The drawing under review shows one solid part. Ordinate dimensions are in mm from its lowest x, y, z. A direction names the side the tool comes from. Give positions to 0.01 mm unless a question says otherwise; leave off trailing zeros. Write each loop counter-clockwise with the first axis right and the second up, starting at its lowest first coordinate (ties: lowest second). Pieces come first, ordered by that corner, then holes. Notation, with made-up numbers: M 89,-25 L 125,-25 A32 cw 125,10 Z; hole C 76,76 d8. An arc over 180 degrees is marked long. Write item = value, one per line. Start each with the question number.
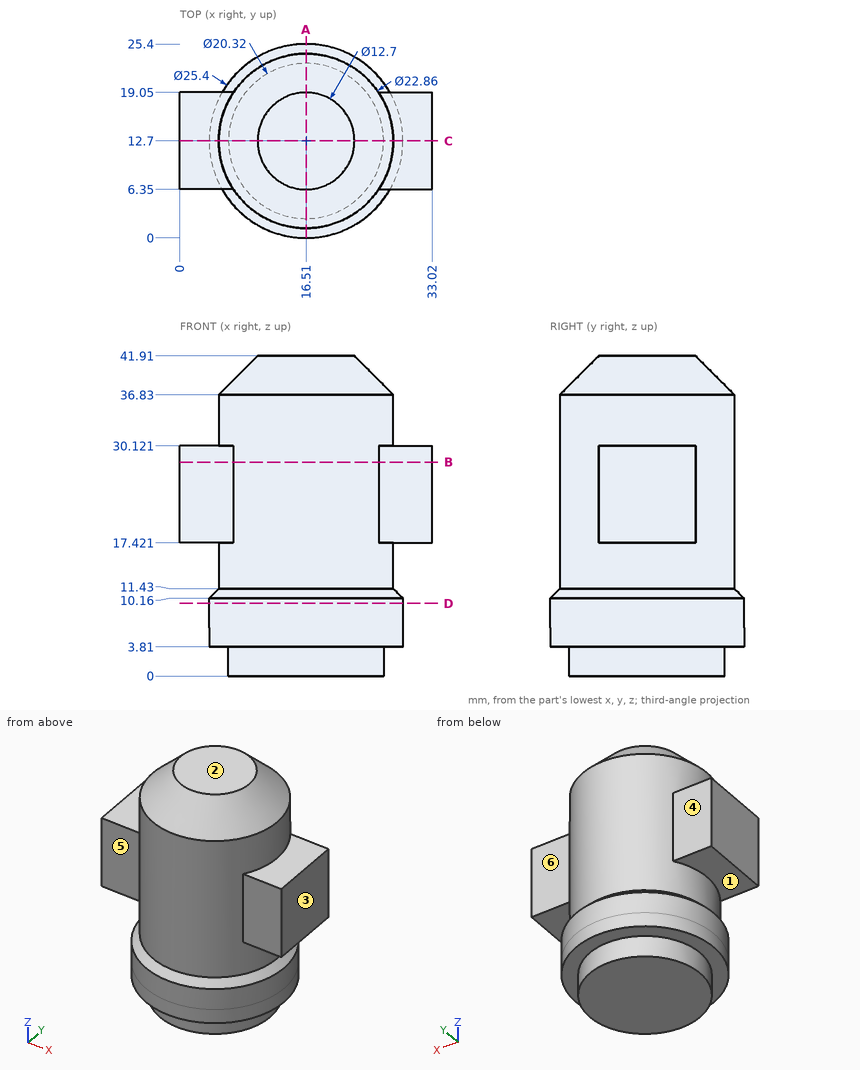
Item 1: We need section C-C, the plane y = 12.7. Write out the cut boundary in (x, z).
Item 2: To check wall thickness, follow probe 1 along Z at (x, y) = (4, 16.75); probe 2 along Y at (x, z) = (4, 18); probe 3 along Z at (x, y) = (5, 9.5). State the ranges of each line that lie inside material, in increasing order. Write a range as [from, to].
Item 3: For the marked faces 4, 5 and 6, list the 3-axis set-ups (+Z, -Z, +X, -X, +Y, -Y) from which the entire face can be reached by the end or side of a thin tool; tool diameter is ignored.
Item 4: Clearance check with flat-ended pins moving along their axes: P1, Ø10, axis at x = 25, z = 35, coming from the -Y side; P2, Ø6, axis at x = 6, y = 4, coming from the +Z side; P3, Ø7.5, axis at x = 4, y = 15.5, coming from the -Z side; P4, Ø5.5, axis at x = 29.5, z = 24, coming from the -Y side. State where each tip first meets the part, or that it passes through.
Item 5: The part is to be moulded in two halves that separate along Z. For the marked faces 1, 2 and 3, say which applies: released by +Z, released by -Z, zero draft, split by the parting line, or undercut.
Item 6: We need section D-D, the plane z = 9.5. Write out the cut boundary in (x, y), and give its area (3 significant figures).
Item 7: We need section A-A, the plane x = 16.51. Write out the cut boundary in (y, z), and give its area (3 significant figures).
Item 8: We need section B-B, the plane z = 28. Write out the cut boundary in (x, y).
Worked out:
q1.outline = M 0,17.42 L 5.08,17.42 L 5.08,11.43 L 3.81,10.16 L 3.81,3.81 L 6.35,3.81 L 6.35,0 L 26.67,0 L 26.67,3.81 L 29.21,3.81 L 29.21,10.16 L 27.94,11.43 L 27.94,17.42 L 33.02,17.42 L 33.02,30.12 L 27.94,30.12 L 27.94,36.83 L 22.86,41.91 L 10.16,41.91 L 5.08,36.83 L 5.08,30.12 L 0,30.12 Z
q2.probe_1 = [17.42, 30.12]
q2.probe_2 = [6.35, 19.05]
q2.probe_3 = [3.81, 10.91], [17.42, 30.12]
q3.face_4 = +Z, -X, +Y
q3.face_5 = +Z, -X, -Y
q3.face_6 = +Z, +X, +Y
q4.P1 = 1.82
q4.P2 = 37.62
q4.P3 = 0
q4.P4 = 6.35
q5.face_1 = undercut
q5.face_2 = released by +Z
q5.face_3 = zero draft
q6.outline = C 16.51,12.7 d25.4
q6.area = 507 mm²
q7.outline = M 0,3.81 L 2.54,3.81 L 2.54,0 L 22.86,0 L 22.86,3.81 L 25.4,3.81 L 25.4,10.16 L 24.13,11.43 L 24.13,36.83 L 19.05,41.91 L 6.35,41.91 L 1.27,36.83 L 1.27,11.43 L 0,10.16 Z
q7.area = 940 mm²
q8.outline = M 0,6.35 L 7.01,6.35 A11.43 ccw 26.01,6.35 L 33.02,6.35 L 33.02,19.05 L 26.01,19.05 A11.43 ccw 7.01,19.05 L 0,19.05 Z
